Check sheet for the modelled part. Datum: model origin and axes. Units: mm. Coordinates: 2 decimals unless noted, no trailing zeros. Loops run counter-clockwise (first coordinate to the right, second up) from the corner with the lowest first, then second, coordinate; pieces in that order, holes last. Notation, with made-up numbers: (68.25, 53) -> (85.25, 53) arc R19 ccw to (85.25, 81) -> close; hole circle Ø3 at (-35.75, 83.25). An arc over 180 degrees is marked (long way). Use CSV: the item, a comma, the result in double quotes.
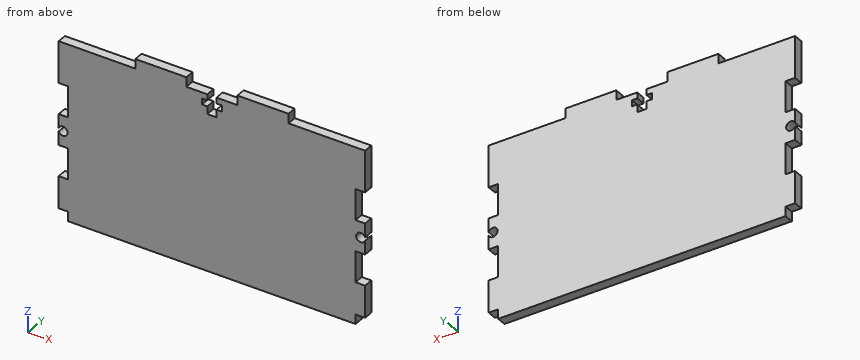
```python
from build123d import *

# Parameters (mm, degrees)
SKETCH2_W           = 96.52
SKETCH2_H           = 55.42
BOSS_EXTRUDE1_DEPTH = 3
SKETCH3_W           = 29.21
SKETCH3_H           = 3
CUT_EXTRUDE1_DEPTH  = 3
SKETCH5_W           = 48.26
SKETCH5_H           = 3
BOSS_EXTRUDE2_DEPTH = 3
SKETCH14_W          = 16.086666666
SKETCH14_H          = 3
CUT_EXTRUDE2_DEPTH  = 3
SKETCH15_W          = 9.737913064
SKETCH15_H          = 3
BOSS_EXTRUDE9_DEPTH = 3
SKETCH26_W          = 3
SKETCH26_H          = 3
CUT_EXTRUDE4_DEPTH  = 3
CUT_EXTRUDE5_DEPTH  = 3
SKETCH29_W          = 2.9
SKETCH29_H          = 3
CUT_EXTRUDE6_DEPTH  = 6.2
SKETCH30_W          = 6.27
SKETCH30_H          = 1.926429006
CUT_EXTRUDE7_DEPTH  = 3


with BuildPart() as part:
    # Sketch2 → Boss-Extrude1 (new body)
    with BuildSketch(Plane(origin=(0, 0, 0), x_dir=(1, 0, 0), z_dir=(0, 1, 0))):
        Rectangle(SKETCH2_W, SKETCH2_H)
    extrude(amount=BOSS_EXTRUDE1_DEPTH)

    # Sketch3 → Cut-Extrude1 (cut)
    with BuildSketch(Plane.ZY.offset(48.26)):
        with Locations((0, 1.5)):
            Rectangle(SKETCH3_W, SKETCH3_H)
    cut_extrude1 = extrude(amount=-CUT_EXTRUDE1_DEPTH, mode=Mode.SUBTRACT)

    # Mirror1: Cut-Extrude1 across plane
    add(cut_extrude1.mirror(Plane(origin=(0, 0, 0), x_dir=(0, 0, 1), z_dir=(1, 0, 0))), mode=Mode.SUBTRACT)

    # Sketch5 → Boss-Extrude2 (add)
    with BuildSketch(Plane.XY.offset(27.71)):
        with Locations((0, 1.5)):
            Rectangle(SKETCH5_W, SKETCH5_H)
    extrude(amount=BOSS_EXTRUDE2_DEPTH)

    # Sketch14 → Cut-Extrude2 (cut)
    with BuildSketch(Plane.XY.offset(30.71)):
        with Locations((0, 1.5)):
            Rectangle(SKETCH14_W, SKETCH14_H)
    extrude(amount=-CUT_EXTRUDE2_DEPTH, mode=Mode.SUBTRACT)

    # Sketch15 → Boss-Extrude9 (add)
    with BuildSketch(Plane(origin=(45.26, 0, 0), x_dir=(0, 0, -1), z_dir=(1, 0, 0))):
        with Locations((0, 1.5)):
            Rectangle(SKETCH15_W, SKETCH15_H)
    boss_extrude9 = extrude(amount=BOSS_EXTRUDE9_DEPTH)

    # Mirror2: Boss-Extrude9 across plane
    add(boss_extrude9.mirror(Plane(origin=(0, 0, 0), x_dir=(0, 0, 1), z_dir=(1, 0, 0))))

    # Sketch26 → Cut-Extrude4 (cut)
    with BuildSketch(Plane(origin=(0, 0, -27.71), x_dir=(-1, 0, 0), z_dir=(0, 0, -1))):
        with Locations((-46.76, 1.5)):
            Rectangle(SKETCH26_W, SKETCH26_H)
    cut_extrude4 = extrude(amount=-CUT_EXTRUDE4_DEPTH, mode=Mode.SUBTRACT)

    # Mirror3: Cut-Extrude4 across plane
    add(cut_extrude4.mirror(Plane(origin=(0, 0, 0), x_dir=(0, 0, 1), z_dir=(1, 0, 0))), mode=Mode.SUBTRACT)

    # Sketch27 → Cut-Extrude5 (cut)
    with BuildSketch(Plane.XZ):
        with BuildLine():
            ThreePointArc((48.26, -0.546659717), (48.334780685, -0.286767695), (48.36, -0.017509454))
            ThreePointArc((48.36, -0.017509454), (48.334780685, 0.251748786), (48.26, 0.511640808))
            Line((48.26, 0.511640808), (48.26, -0.546659717))
        make_face()
        with BuildLine():
            Line((48.26, -0.546659717), (48.26, 0.511640808))
            ThreePointArc((48.26, 0.511640808), (45.46, -0.017509454), (48.26, -0.546659717))
        make_face()
    cut_extrude5 = extrude(amount=-CUT_EXTRUDE5_DEPTH, mode=Mode.SUBTRACT)

    # Mirror4: Cut-Extrude5 across plane
    add(cut_extrude5.mirror(Plane(origin=(0, 0, 0), x_dir=(0, 0, 1), z_dir=(1, 0, 0))), mode=Mode.SUBTRACT)

    # Sketch29 → Cut-Extrude6 (cut)
    with BuildSketch(Plane.XY.offset(27.71)):
        with Locations((0, 1.5)):
            Rectangle(SKETCH29_W, SKETCH29_H)
    extrude(amount=-CUT_EXTRUDE6_DEPTH, mode=Mode.SUBTRACT)

    # Sketch30 → Cut-Extrude7 (cut)
    with BuildSketch(Plane.XZ):
        with Locations((0, 24.88885073)):
            Rectangle(SKETCH30_W, SKETCH30_H)
    extrude(amount=-CUT_EXTRUDE7_DEPTH, mode=Mode.SUBTRACT)


solid = part.part
```
1) Go/stop test with flat-tipped pins: pin 1 Ø1.4 at (x, y) = (0.5, 1) entering from +Z; pin 2 Ø0.9 at (x, y) = (46.5, 1) entering from -Z; pin 3 Ø4 at (x, z) = (46.91, -0.02) entering from +Y; pin 4 Ø0.9 at (y, z) = (1, 30) entering from +X. Record where each tip stops, or that it passes through.
Answer below:
pin 1,"stops at z = 21.51"
pin 2,"stops at z = -24.71"
pin 3,"stops at y = 3"
pin 4,"stops at x = 24.13"
2) Cross-section at A-A on x = 46.91. Record the boundary of the cut face in (y, z) (1 decimal), and give its area (3 significant figures).
Answer below:
outline,"(0, -24.7) -> (3, -24.7) -> (3, -14.6) -> (0, -14.6) -> close; (0, -4.9) -> (3, -4.9) -> (3, -1.5) -> (0, -1.5) -> close; (0, 1.4) -> (3, 1.4) -> (3, 4.9) -> (0, 4.9) -> close; (0, 14.6) -> (3, 14.6) -> (3, 27.7) -> (0, 27.7) -> close"
area,"90.1 mm²"
3) Thickness scan on line 1 along Z through (x, y) = (46.91, 2.15) (1 decimal); line 2 along X through (y, z) = (0.6, 24) (3 decimals); line 3 along Z through (x, y) = (-28, 1.8). Record the ranges inside material, lowest first. Write a range as from..to.
Answer below:
line 1,"z = -24.7..-14.6, -4.9..-1.5, 1.4..4.9, 14.6..27.7"
line 2,"x = -48.26..-3.135, 3.135..48.26"
line 3,"z = -27.71..27.71"
4) Cross-section at B-B on z = 9. Record the boundary of the cut face in (x, y), and give its area (3 significant figures).
Answer below:
outline,"(-45.26, 0) -> (45.26, 0) -> (45.26, 3) -> (-45.26, 3) -> close"
area,"272 mm²"
